Input: part model. Units: mm. Frame: model coordinates. A direction names the side the tool comes from. Round coordinates to 2 decimals unless told otherwise and drop trailing zeros. Loops run counter-clockwise (first coordinate to the right, second up) from the corner with the lowest first, then second, coordinate; pieces in that order, holes last. Notation, with made-up numbers: (1, 19) -> (30, 19) arc R21 ccw to (30, 33) -> close; hole circle Ø5 at (15.25, 59). An arc over 180 degrees is marked (long way). Answer as a JSON object with one key per item and string values. Group by question number.
Item 1: Section query A-A on z = 29.21. Count the separate pieces of the cut face and the enclosed holes in it, and give its area (3 significant figures).
Item 2: Set-up query: faces 1 (the flat face through (36.83, 16, -34)), 2 (the flat face through (-11, 32, -10.5)). Return all of +Z, -Z, +X, -X, +Y, -Y with unobstructed straight access to the full face (end or side cutting, diameter ignored); none if empty.
Item 3: Pin query (flat end, axial travel): pin 1 (1.5 mm diameter, centred on x = -11.5, z = 17.5, fed in from -Y); pin 2 (3 mm diameter, centred on y = 33.5, z = 6, fed in from -X); pin 3 (8 mm diameter, centred on x = 52.5, y = 8.5, fed in from -Z). Return the tip coordinate at first contact, or that it passes through.
Item 4: Section query C-C on x = 29.21. Return loops of the section in (y, z).
Item 5: Draft query along Z for faces 3 (the flat face through (-26.67, 16, 15)), 4 (the flat face through (-15, 0, 46)). Return one class per face: released by +Z, released by -Z, zero draft, split by the parting line, or undercut.
Item 6: Material intervals for line 1 (X direction, y = 27, z = 29); line 2 (Z direction, x = 34, y = 21.5); line 3 (X direction, y = 21.5, z = -13.5), sorted ascending. Write a range as [from, to].
from build123d import *

# Parameters (mm, degrees)
EXTRUDE_THIN1_DEPTH     = 50.8
CUT_EXTRUDE1_REACH      = 92.098
SKETCH4_W               = 25.4
SKETCH4_H               = 19.05
FILLET1_R               = 2.54
EXTRUDE_THIN2_REACH     = 92.098
SKETCH3_W               = 63.5
SKETCH3_H               = 2.54
SKETCH9_W               = 2.54
SKETCH9_H               = 38.1
SKETCH9_H_2             = 91.44
SKETCH9_H_3             = 24.13
EXTRUDE_THIN3_DEPTH     = 31.75
CUT_EXTRUDE2_REACH      = 92.098
SKETCH5_W               = 42.5
SKETCH5_H               = 21
M4_CLEARANCE_HOLE1_D    = 4.8
CUT_EXTRUDE4_REACH      = 92.098
SKETCH7_W               = 7.96
SKETCH7_H               = 2.032
CUT_EXTRUDE5_REACH      = 113.138
SKETCH10_W              = 12.7
SKETCH10_H              = 9.525
M3_CLEARANCE_HOLE1_D    = 3.6
M8_CLEARANCE_HOLE1_D    = 10
SKETCH19_W              = 102.87
SKETCH19_H              = 72.39
SKETCH19_W_2            = 92.71
SKETCH19_H_2            = 62.23
CUT_EXTRUDE_THIN1_DEPTH = 2.54


# Read off the part's stored shape, not the designer's step: Mirror2
with BuildPart() as part:
    # Sketch2 → Extrude-Thin1 (new, symmetric)
    with BuildSketch(Plane.XY):
        Polygon((0, 31.75), (63.5, 31.75), (63.5, 0), (66.04, 0), (66.04, 34.29), (0, 34.29), align=None)
    extrude(amount=EXTRUDE_THIN1_DEPTH, both=True)

    # Sketch4 → Cut-Extrude1 (cut, up to next)
    with BuildSketch(Plane(origin=(66.04, 0, 0), x_dir=(0, 0, -1), z_dir=(1, 0, 0)), mode=Mode.PRIVATE) as cut_extrude1_sk1:
        with Locations((0, 9.525)):
            Rectangle(SKETCH4_W, SKETCH4_H)
    cut_extrude1_tool1 = extrude(cut_extrude1_sk1.sketch, amount=-CUT_EXTRUDE1_REACH, mode=Mode.PRIVATE) & part.part
    add(cut_extrude1_tool1.solids().sort_by_distance((66.04, 9.525, 0))[0], mode=Mode.SUBTRACT)

    # Fillet1
    fillet1_edges = [part.edges().sort_by_distance(p)[0] for p in [
        (64.77, 19.05, 12.7),
        (64.77, 19.05, -12.7),
        (63.5, 31.75, 0),
        (66.04, 34.29, 0),
    ]]
    fillet(fillet1_edges, radius=FILLET1_R)

    # Sketch3 → Extrude-Thin2 (add, up to next)
    with BuildSketch(Plane.XZ, mode=Mode.PRIVATE) as extrude_thin2_sk1:
        with Locations((31.75, 20.32)):
            Rectangle(SKETCH3_W, SKETCH3_H)
    extrude_thin2_tool1 = extrude(extrude_thin2_sk1.sketch, amount=-EXTRUDE_THIN2_REACH, mode=Mode.PRIVATE) - part.part
    # Sketch3 → Extrude-Thin2 (add, up to next)
    with BuildSketch(Plane.XZ, mode=Mode.PRIVATE) as extrude_thin2_sk2:
        with Locations((31.75, 46.99)):
            Rectangle(SKETCH3_W, SKETCH3_H)
    extrude_thin2_tool2 = extrude(extrude_thin2_sk2.sketch, amount=-EXTRUDE_THIN2_REACH, mode=Mode.PRIVATE) - part.part
    extrude_thin2_1 = extrude_thin2_tool1.solids().sort_by_distance((31.75, 0, 20.32))[0]
    add(extrude_thin2_1)
    extrude_thin2_2 = extrude_thin2_tool2.solids().sort_by_distance((31.75, 0, 46.99))[0]
    add(extrude_thin2_2)
    extrude_thin2 = extrude_thin2_1 + extrude_thin2_2  # Extrude-Thin2 as one shape, for the pattern or mirror that repeats it

    # Mirror1: Extrude-Thin2 across plane
    add(extrude_thin2.mirror(Plane.XY))

    # Mirror2: part across plane


with BuildPart() as part_1:
    add(part.part)
    add(part.part.mirror(Plane(origin=(0, 0, 0), x_dir=(0, 0, 1), z_dir=(1, 0, 0))))

    # Sketch9 → Extrude-Thin3 (add)
    with BuildSketch(Plane.XZ):
        with Locations((-25.4, 0)):
            Rectangle(SKETCH9_W, SKETCH9_H)
        Rectangle(SKETCH9_W, SKETCH9_H_2)
        with Locations((25.4, 0)):
            Rectangle(SKETCH9_W, SKETCH9_H)
        with Locations((-35.56, 33.655)):
            Rectangle(SKETCH9_W, SKETCH9_H_3)
        with Locations((-35.56, -33.655)):
            Rectangle(SKETCH9_W, SKETCH9_H_3)
        with Locations((35.56, 33.655)):
            Rectangle(SKETCH9_W, SKETCH9_H_3)
        with Locations((35.56, -33.655)):
            Rectangle(SKETCH9_W, SKETCH9_H_3)
    extrude(amount=-EXTRUDE_THIN3_DEPTH)

    # Sketch5 → Cut-Extrude2 (cut, up to next)
    with BuildSketch(Plane(origin=(0, 34.29, 0), x_dir=(1, 0, 0), z_dir=(0, 1, 0)), mode=Mode.PRIVATE) as cut_extrude2_sk1:
        with Locations((-9.464, 0)):
            Rectangle(SKETCH5_W, SKETCH5_H)
    cut_extrude2_tool1 = extrude(cut_extrude2_sk1.sketch, amount=-CUT_EXTRUDE2_REACH, mode=Mode.PRIVATE) & part_1.part
    add(cut_extrude2_tool1.solids().sort_by_distance((-9.464, 34.29, 0))[0], mode=Mode.SUBTRACT)

    # M4 Clearance Hole1 (through all)
    with Locations(Plane(origin=(0, 34.29, 0), x_dir=(1, 0, 0), z_dir=(0, 1, 0))):
        with Locations((15.286, -5), (15.286, 5), (-34.214, 5), (-34.214, -5)):
            Hole(M4_CLEARANCE_HOLE1_D / 2)

    # Sketch7 → Cut-Extrude4 (cut, up to next)
    with BuildSketch(Plane(origin=(0, 34.29, 0), x_dir=(1, 0, 0), z_dir=(0, 1, 0)), mode=Mode.PRIVATE) as cut_extrude4_sk1:
        with Locations((15.766, 0)):
            Rectangle(SKETCH7_W, SKETCH7_H)
    cut_extrude4_tool1 = extrude(cut_extrude4_sk1.sketch, amount=-CUT_EXTRUDE4_REACH, mode=Mode.PRIVATE) & part_1.part
    # Sketch7 → Cut-Extrude4 (cut, up to next)
    with BuildSketch(Plane(origin=(0, 34.29, 0), x_dir=(1, 0, 0), z_dir=(0, 1, 0)), mode=Mode.PRIVATE) as cut_extrude4_sk2:
        with Locations((-34.694, 0)):
            Rectangle(SKETCH7_W, SKETCH7_H)
    cut_extrude4_tool2 = extrude(cut_extrude4_sk2.sketch, amount=-CUT_EXTRUDE4_REACH, mode=Mode.PRIVATE) & part_1.part
    add(cut_extrude4_tool1.solids().sort_by_distance((15.766, 34.29, 0))[0], mode=Mode.SUBTRACT)
    add(cut_extrude4_tool2.solids().sort_by_distance((-34.694, 34.29, 0))[0], mode=Mode.SUBTRACT)

    # Sketch10 → Cut-Extrude5 (cut, up to next)
    with BuildSketch(Plane(origin=(26.67, 0, 0), x_dir=(0, 0, -1), z_dir=(1, 0, 0)), mode=Mode.PRIVATE) as cut_extrude5_sk1:
        with Locations((0, 4.7625)):
            Rectangle(SKETCH10_W, SKETCH10_H)
    cut_extrude5_tool1 = extrude(cut_extrude5_sk1.sketch, amount=-CUT_EXTRUDE5_REACH, mode=Mode.PRIVATE) & part_1.part
    add(cut_extrude5_tool1.solids().sort_by_distance((26.67, 4.7625, 0))[0], mode=Mode.SUBTRACT)

    # M3 Clearance Hole1 (through all)
    with Locations(Plane(origin=(0, 34.29, 0), x_dir=(1, 0, 0), z_dir=(0, 1, 0))):
        with Locations((-29.21, 29.21), (29.21, 29.21), (29.21, -29.21), (-29.21, -29.21)):
            Hole(M3_CLEARANCE_HOLE1_D / 2)

    # M8 Clearance Hole1 (through all)
    with Locations(Plane(origin=(0, 34.29, 0), x_dir=(1, 0, 0), z_dir=(0, 1, 0))):
        with Locations((41.309178157, 0)):
            Hole(M8_CLEARANCE_HOLE1_D / 2)

    # Sketch19 → Cut-Extrude-Thin1 (cut)
    with BuildSketch(Plane(origin=(0, 0, 0), x_dir=(-1, 0, 0), z_dir=(0, -1, 0))):
        Rectangle(SKETCH19_W, SKETCH19_H)
        Rectangle(SKETCH19_W_2, SKETCH19_H_2, mode=Mode.SUBTRACT)
    extrude(amount=-CUT_EXTRUDE_THIN1_DEPTH, mode=Mode.SUBTRACT)


solid = part_1.part
Solved:
{
 "1": {"separate pieces": "3", "enclosed holes": "0", "area": "720 mm²"},
 "2": {"face 1": "-Y", "face 2": "+Y, -Y"},
 "3": {"pin 1": "y = 31.75", "pin 2": "x = -66.03", "pin 3": "z = -48.26"},
 "4": {"outline": "(0, -48.26) -> (31.75, -48.26) -> (31.75, -50.8) -> (34.29, -50.8) -> (34.29, -31.01) -> (31.75, -31.01) -> (31.75, -45.72) -> (0, -45.72) -> close; (0, -21.59) -> (31.75, -21.59) -> (31.75, -27.41) -> (34.29, -27.41) -> (34.29, 27.41) -> (31.75, 27.41) -> (31.75, 21.59) -> (0, 21.59) -> (0, 19.05) -> (31.75, 19.05) -> (31.75, -19.05) -> (0, -19.05) -> close; (0, 45.72) -> (31.75, 45.72) -> (31.75, 31.01) -> (34.29, 31.01) -> (34.29, 50.8) -> (31.75, 50.8) -> (31.75, 48.26) -> (0, 48.26) -> close"},
 "5": {"face 3": "undercut", "face 4": "zero draft"},
 "6": {"line 1": "[-66.04, -63.5], [-36.83, -34.29], [-1.27, 1.27], [34.29, 36.83], [63.5, 66.04]", "line 2": "[-48.26, -45.72], [-21.59, -19.05], [19.05, 21.59], [45.72, 48.26]", "line 3": "[-66.04, -63.5], [-26.67, -24.13], [-1.27, 1.27], [24.13, 26.67], [63.5, 66.04]"}
}
